```python
from build123d import *

# Parameters (mm, degrees)
F1_DEPTH = 63.5
F2_DEPTH = 25.4
F3_DEPTH = 7.9375


with BuildPart() as f1:
    # F0 (on Front) → F1 (new body, symmetric)
    with BuildSketch(Plane.XZ):
        Polygon((-41.275, 9.525), (-41.275, -9.525), (41.275, -9.525), (41.275, 9.525), (22.225, 9.525), align=None)
    extrude(amount=F1_DEPTH, both=True)

    # F0 (on Front) → F2 (join, symmetric)
    with BuildSketch(Plane.XZ):
        with BuildLine():
            Line((22.225, 9.525), (41.275, 9.525))
            Line((41.275, 9.525), (41.275, 27.0002))
            ThreePointArc((41.275, 27.0002), (45.9246798487, 38.2255201513), (57.15, 42.8752))
            Line((57.15, 42.8752), (60.325, 42.8752))
            Line((60.325, 42.8752), (60.325, 61.9252))
            Line((60.325, 61.9252), (57.15, 61.9252))
            add(Edge.make_bspline(
                [(56.0439940471, 61.9076830922), (56.4136969839, 61.9136063659), (56.7823811234, 61.9194348071), (57.15, 61.9252)],
                knots=[110.5340718473, 110.5340718473, 110.5340718473, 110.5340718473, 111.5045361635, 111.5045361635, 111.5045361635, 111.5045361635], degree=3))
            ThreePointArc((56.0439940471, 61.9076830922), (32.0663112471, 51.3017263625), (22.225, 27.0002))
            Line((22.225, 27.0002), (22.225, 9.525))
        make_face()
        Polygon((60.325, 66.675), (60.325, 61.9252), (60.325, 42.8752), (86.0297148728, 42.8752), (85.725, 66.675), align=None)
    extrude(amount=F2_DEPTH, both=True)

    # F0 (on Front) → F3 (join, symmetric)
    with BuildSketch(Plane.XZ):
        with BuildLine():
            add(Edge.make_bspline(
                [(-41.275, 9.525), (-41.3895917306, 59.328141832), (13.9355205015, 61.2330332862), (56.0439940471, 61.9076830922)],
                knots=[0, 0, 0, 0, 110.5340718473, 110.5340718473, 110.5340718473, 110.5340718473], degree=3))
            Line((-41.275, 9.525), (22.225, 9.525))
            Line((22.225, 9.525), (22.225, 27.0002))
            ThreePointArc((22.225, 27.0002), (32.0663112471, 51.3017263625), (56.0439940471, 61.9076830922))
        make_face()
    extrude(amount=F3_DEPTH, both=True)


solid = f1.part
```
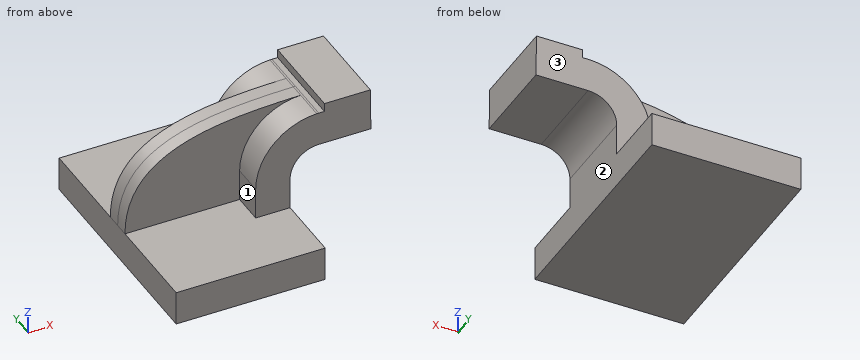
Verification items for the finished model (mm, model axes). Face numbers are marked on the shaded views. A direction names the side the tool comes from. Round coordinates to 2 decimals unless told otherwise and drop trailing zeros. Loops run counter-clockwise (first coordinate to the right, second up) from the corner with the lowest first, then second, coordinate; pieces in that order, holes last. Notation, with made-up numbers: (53, 67) -> (98, 67) arc R12 cw to (98, 75) -> close; hole circle Ø7 at (5.25, -35). An arc over 180 degrees is marked (long way). Answer as a JSON object with one key per item and string values.
Q1. Section check A-A (z = -4). Record the boundary of the cut face in (x, y) (3 decimals), then the cut area to 3 significant figures.
Data:
{"outline": "(-41.275, -63.5) -> (41.275, -63.5) -> (41.275, 63.5) -> (-41.275, 63.5) -> close", "area": "10,500 mm2"}
Q2. Go/stop test with flat-tipped pins: P1, Ø15.5, axis at x = -16, z = 44.5, coming from the -Y side; P2, Ø1, axis at x = 16, z = 49.5, coming from the +Y side; P3, Ø14.5, axis at x = 66, y = 8, coming from the -Z side. Record where each tip stops, or that it passes through.
Data:
{"P1": "stops at y = -7.94", "P2": "stops at y = 7.94", "P3": "stops at z = 42.88"}
Q3. Access from +Z, -Z, +X, -X, +Y, -Y to the whole of each face (thin tool, end or side, straight path). Record for the marked faces 1, 2 and 3.
Data:
{"face 1": "+Z, -X, -Y", "face 2": "-Z, +X, +Y, -Y", "face 3": "+Z, +X, -X, +Y"}
Q4. Section check B-B (y = 43). Record the boundary of the cut face in (x, z) (3 decimals), then the cut area to 3 significant figures.
Data:
{"outline": "(-41.275, -9.525) -> (41.275, -9.525) -> (41.275, 9.525) -> (-41.275, 9.525) -> close", "area": "1,570 mm2"}
Q5. Scan lines: line 1 (X direction, y = -13, z = 20.5) (3 decimals); line 2 (Z direction, x = 3, y = -18.5) (3 decimals); line 3 (Y direction, x = 13, z = 43). Record each from-to range of solid material in increasing order. Write a range as from..to.
Data:
{"line 1": "x = 22.225..41.275", "line 2": "z = -9.525..9.525", "line 3": "y = -7.94..7.94"}
